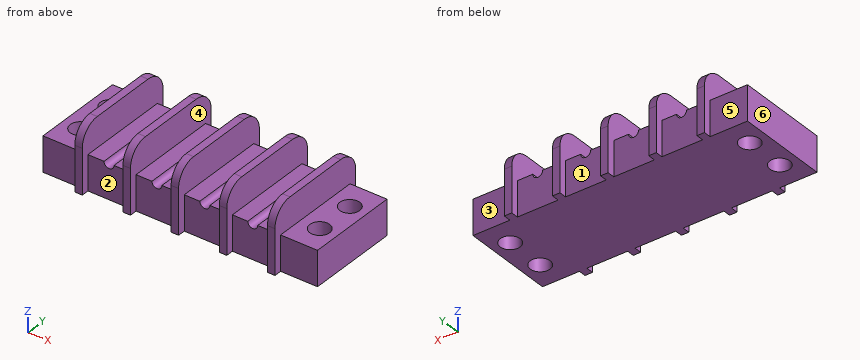
```python
from build123d import *

# Parameters (mm, degrees)
ESQUISSE1_W                = 55
ESQUISSE1_H                = 18.5
BOSS_EXTRU_1_DEPTH         = 7
ENL_V_MAT_EXTRU_1_REACH    = 9
ESQUISSE2_R                = 2
ESQUISSE3_W                = 1.5
ESQUISSE3_H                = 21.5
BOSS_EXTRU_2_DEPTH         = 13
CONG_1_R                   = 4
ESQUISSE4_R                = 1
ENL_V_MAT_EXTRU_2_DEPTH    = 18.5
R_P_TITION_LIN_AIRE1_COUNT = 4
R_P_TITION_LIN_AIRE1_PITCH = 9.6


with BuildPart() as part:
    # Esquisse1 → Boss.-Extru.1 (new body)
    with BuildSketch(Plane.XY):
        with Locations((-1.745283019, 3.839622642)):
            Rectangle(ESQUISSE1_W, ESQUISSE1_H)
    extrude(amount=BOSS_EXTRU_1_DEPTH)

    # Esquisse2 → Enlèv. mat.-Extru.1 (cut, up to next)
    with BuildSketch(Plane(origin=(0, 0, 0), x_dir=(-1, 0, 0), z_dir=(0, 0, -1)), mode=Mode.PRIVATE) as enl_v_mat_extru_1_sk1:
        with Locations((-22.254716981, 7.839622642)):
            Circle(ESQUISSE2_R)
    enl_v_mat_extru_1_tool1 = extrude(enl_v_mat_extru_1_sk1.sketch, amount=-ENL_V_MAT_EXTRU_1_REACH, mode=Mode.PRIVATE) & part.part
    add(enl_v_mat_extru_1_tool1.solids().sort_by_distance((22.254717, 7.839623, 0))[0], mode=Mode.SUBTRACT)
    # Esquisse2 → Enlèv. mat.-Extru.1 (cut, up to next)
    with BuildSketch(Plane(origin=(0, 0, 0), x_dir=(-1, 0, 0), z_dir=(0, 0, -1)), mode=Mode.PRIVATE) as enl_v_mat_extru_1_sk2:
        with Locations((-22.254716981, -0.160377358)):
            Circle(ESQUISSE2_R)
    enl_v_mat_extru_1_tool2 = extrude(enl_v_mat_extru_1_sk2.sketch, amount=-ENL_V_MAT_EXTRU_1_REACH, mode=Mode.PRIVATE) & part.part
    add(enl_v_mat_extru_1_tool2.solids().sort_by_distance((22.254717, -0.160377, 0))[0], mode=Mode.SUBTRACT)
    # Esquisse2 → Enlèv. mat.-Extru.1 (cut, up to next)
    with BuildSketch(Plane(origin=(0, 0, 0), x_dir=(-1, 0, 0), z_dir=(0, 0, -1)), mode=Mode.PRIVATE) as enl_v_mat_extru_1_sk3:
        with Locations((25.745283019, -0.160377358)):
            Circle(ESQUISSE2_R)
    enl_v_mat_extru_1_tool3 = extrude(enl_v_mat_extru_1_sk3.sketch, amount=-ENL_V_MAT_EXTRU_1_REACH, mode=Mode.PRIVATE) & part.part
    add(enl_v_mat_extru_1_tool3.solids().sort_by_distance((-25.745283, -0.160377, 0))[0], mode=Mode.SUBTRACT)
    # Esquisse2 → Enlèv. mat.-Extru.1 (cut, up to next)
    with BuildSketch(Plane(origin=(0, 0, 0), x_dir=(-1, 0, 0), z_dir=(0, 0, -1)), mode=Mode.PRIVATE) as enl_v_mat_extru_1_sk4:
        with Locations((25.745283019, 7.839622642)):
            Circle(ESQUISSE2_R)
    enl_v_mat_extru_1_tool4 = extrude(enl_v_mat_extru_1_sk4.sketch, amount=-ENL_V_MAT_EXTRU_1_REACH, mode=Mode.PRIVATE) & part.part
    add(enl_v_mat_extru_1_tool4.solids().sort_by_distance((-25.745283, 7.839623, 0))[0], mode=Mode.SUBTRACT)

    # Esquisse3 → Boss.-Extru.2 (add)
    with BuildSketch(Plane(origin=(0, 0, 0), x_dir=(-1, 0, 0), z_dir=(0, 0, -1))):
        with Locations((20.995283019, 3.839622642)):
            Rectangle(ESQUISSE3_W, ESQUISSE3_H)
        with Locations((11.345283019, 3.839622642)):
            Rectangle(ESQUISSE3_W, ESQUISSE3_H)
        with Locations((1.695283019, 3.839622642)):
            Rectangle(ESQUISSE3_W, ESQUISSE3_H)
        with Locations((-7.954716981, 3.839622642)):
            Rectangle(ESQUISSE3_W, ESQUISSE3_H)
        with Locations((-17.604716981, 3.839622642)):
            Rectangle(ESQUISSE3_W, ESQUISSE3_H)
    extrude(amount=-BOSS_EXTRU_2_DEPTH)

    # Congé1
    cong_1_edges = [part.edges().sort_by_distance(p)[0] for p in [
        (17.604716981, -6.910377358, 13),
        (17.604716981, 14.589622642, 13),
        (-20.995283019, -6.910377358, 13),
        (-20.995283019, 14.589622642, 13),
        (-11.345283019, -6.910377358, 13),
        (-11.345283019, 14.589622642, 13),
        (-1.695283019, -6.910377358, 13),
        (-1.695283019, 14.589622642, 13),
        (7.954716981, -6.910377358, 13),
        (7.954716981, 14.589622642, 13),
    ]]
    fillet(cong_1_edges, radius=CONG_1_R)

    # Esquisse4 → Enlèv. mat.-Extru.2 (cut)
    with BuildSketch(Plane.XZ.offset(5.410377358)):
        with Locations((12.779716981, 7)):
            Circle(ESQUISSE4_R)
    enl_v_mat_extru_2 = extrude(amount=-ENL_V_MAT_EXTRU_2_DEPTH, mode=Mode.SUBTRACT)

    # Répétition linéaire1: Enlèv. mat.-Extru.2 ×4
    with Locations(*[(-i * R_P_TITION_LIN_AIRE1_PITCH, 0, 0) for i in range(1, R_P_TITION_LIN_AIRE1_COUNT)]):
        add(enl_v_mat_extru_2, mode=Mode.SUBTRACT)


solid = part.part
```
Geometry: final body of the model. Coordinates: model frame, mm. Face numbers are marked on the shaded views. A direction names the side the tool comes from. Coordinates: 2 decimals unless noted, no trailing zeros. Order: outer loops, then holes, each group sorted by start corner. A loop starts at its lowest first (then second) coordinate and runs counter-clockwise, first axis right, second up. Notation, with made-up numbers: (78, 23.5) -> (85, 23.5) arc R33 ccw to (85, 53.5) -> close; hole circle Ø8 at (2, 30.25). An arc over 180 degrees is marked (long way). Write each question's results on one line, items separated by ' | '. Start each with the question number.
1) Cut plane B-B, the plane y = 6.75. State how many separate pieces and enclosed holes the cut face has, and give its area (3 significant figures).
2) Cut plane D-D, the plane x = 5. Output: boundary loops of the cut face in (y, z), and give its area (4 significant figures).
3) Mould query, pull axis X, two halves, no side actions, for the marked faces 4, 5 and 6. Classes: released by +X, released by -X, zero draft, split by the parting line, or undercut.
4) Cut plane C-C, the plane z = 12. Output: boundary loops of the cut face in (x, y).
5) Set-up query: the marked faces 1, 2 and 3. Return all of +Z, -Z, +X, -X, +Y, -Y with unobstructed straight access to the full face (end or side cutting, diameter ignored); none if empty.
6) Cut plane A-A, the plane z = 9.5. Output: boundary loops of the cut face in (x, y).
7) First-contact query: pin 1 (5 mm diameter, centred on x = -16, y = 6.5, fed in from -Z); pin 2 (2 mm diameter, centred on x = -25.5, y = 7, fed in from +Z); pin 3 (2.5 mm diameter, centred on x = 15.5, y = 7, fed in from +Z); pin 4 (2 mm diameter, centred on x = -17, z = 4, fed in from -Y). Flat tips, straight axial feed; report the tip coordinate or a pass-through.
8) Material intervals for line 1 along X through (y, z) = (-0.5, 7.5); line 2 along Y through (x, z) = (23, 3.5); line 3 along X through (y, z) = (-1, 2.25), sorted ascending.
Checks:
1) separate pieces: 3 | enclosed holes: 0 | area: 377 mm^2
2) outline: (-5.41, 0) -> (13.09, 0) -> (13.09, 7) -> (-5.41, 7) -> close | area: 129.5 mm^2
3) face 4: undercut | face 5: zero draft | face 6: released by -X
4) outline: (-21.75, -5.56) -> (-20.25, -5.56) -> (-20.25, 13.24) -> (-21.75, 13.24) -> close; (-12.1, -5.56) -> (-10.6, -5.56) -> (-10.6, 13.24) -> (-12.1, 13.24) -> close; (-2.45, -5.56) -> (-0.95, -5.56) -> (-0.95, 13.24) -> (-2.45, 13.24) -> close; (7.2, -5.56) -> (8.7, -5.56) -> (8.7, 13.24) -> (7.2, 13.24) -> close; (16.85, -5.56) -> (18.35, -5.56) -> (18.35, 13.24) -> (16.85, 13.24) -> close
5) face 1: +Z, -Z, +Y | face 2: +Z, -Z, -Y | face 3: +Z, -Z, +X, +Y
6) outline: (-21.75, -6.88) -> (-20.25, -6.88) -> (-20.25, 14.56) -> (-21.75, 14.56) -> close; (-12.1, -6.88) -> (-10.6, -6.88) -> (-10.6, 14.56) -> (-12.1, 14.56) -> close; (-2.45, -6.88) -> (-0.95, -6.88) -> (-0.95, 14.56) -> (-2.45, 14.56) -> close; (7.2, -6.88) -> (8.7, -6.88) -> (8.7, 14.56) -> (7.2, 14.56) -> close; (16.85, -6.88) -> (18.35, -6.88) -> (18.35, 14.56) -> (16.85, 14.56) -> close
7) pin 1: z = 0 | pin 2: through | pin 3: z = 7 | pin 4: y = -5.41
8) line 1: -21.75 to -20.25, -12.1 to -10.6, -2.45 to -0.95, 7.2 to 8.7, 16.85 to 18.35 | line 2: -5.41 to -2.02, 1.7 to 5.98, 9.7 to 13.09 | line 3: -29.25 to -27.56, -23.93 to 20.44, 24.07 to 25.75
